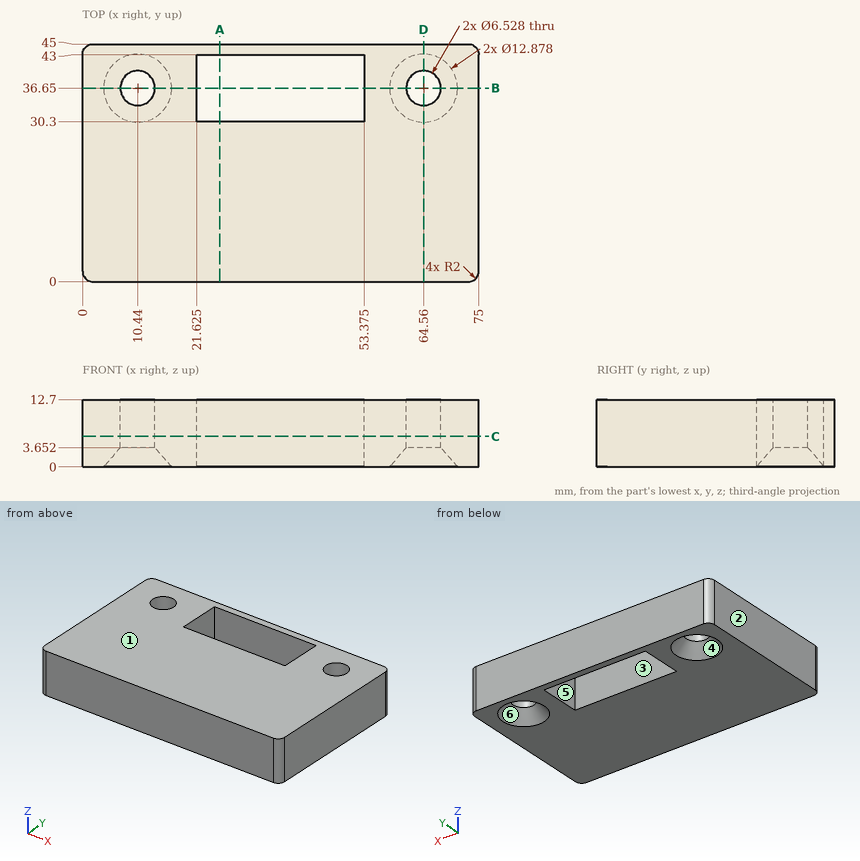
Design review of the part shown in the three views and the two pictorial views. Dimensions are in mm from the part's minimum x, y and z. A direction names the side the tool comes from. Round coordinates to 2 decimals unless told otherwise and drop trailing zeros. Order: outer loops, then holes, each group sorted by start corner. A loop starts at its lowest first (then second) coordinate and runs counter-clockwise, first axis right, second up. Notation, with made-up numbers: (44.25, -9) -> (79.25, -9) arc R18 cw to (79.25, 2) -> close; hole circle Ø8 at (85.25, 59.5). An arc over 180 degrees is marked (long way). Write item = value, one per line. Start each with the question number.
1) Tool access review of the marked faces 5 and 6: name each direction out of +Z, -Z, +X, -X, +Y, -Y from which nothing blocks a thin tool from reaching the whole face with its end or side.
2) Take a section at D-D on x = 64.56. State the section outline as (y, z) points.
3) Insertion check: pin 1 (6 mm diameter, centred on x = 64.56, y = 36.65, fed in from +Z). The pin has a flat end and moves straight along its axis. Give the tip position at first contact, or say it passes through.
4) To check wall thickness, follow line 1 (X direction, y = 36.65, z = 10.75) (1 decimal); line 2 (Y direction, x = 10.44, z = 9); line 3 (Y direction, x = 23, z = 1). State the ranges of each line that lie inside material, in increasing order. Write a range as from..to.
5) Take a section at C-C on z = 5.75. Count the separate pieces of the cut face and the enclosed holes in it, plus the area to 3 significant figures.
6) Take a section at B-B on y = 36.65. State the section outline as (x, z) points (1 decimal).
7) The part is to be moulded in two halves that separate along X. For the marked faces 1, 2, 3 and 4, say which applies: +X half, -X half, draft (parallel to the pull), parting line (faces both ways), or undercut.
8) Take a section at A-A on x = 26. State the section outline as (y, z) points, plus the area to 3 significant figures.
Verdict:
q1.face_5 = +Z, -Z
q1.face_6 = -Z
q2.outline = (0, 0) -> (30.21, 0) -> (33.39, 3.65) -> (33.39, 12.7) -> (0, 12.7) -> close; (39.91, 3.65) -> (43.09, 0) -> (45, 0) -> (45, 12.7) -> (39.91, 12.7) -> close
q3.pin_1 = through
q4.line_1 = 0..7.2, 13.7..21.6, 53.4..61.3, 67.8..75
q4.line_2 = 0..33.39, 39.91..45
q4.line_3 = 0..30.3, 43..45
q5.separate_pieces = 1
q5.enclosed_holes = 3
q5.area = 2,900 mm2
q6.outline = (0, 0) -> (4, 0) -> (7.2, 3.7) -> (7.2, 12.7) -> (0, 12.7) -> close; (13.7, 3.7) -> (16.9, 0) -> (21.6, 0) -> (21.6, 12.7) -> (13.7, 12.7) -> close; (53.4, 0) -> (58.1, 0) -> (61.3, 3.7) -> (61.3, 12.7) -> (53.4, 12.7) -> close; (67.8, 3.7) -> (71, 0) -> (75, 0) -> (75, 12.7) -> (67.8, 12.7) -> close
q7.face_1 = draft
q7.face_2 = -X half
q7.face_3 = undercut
q7.face_4 = undercut
q8.outline = (0, 0) -> (30.3, 0) -> (30.3, 12.7) -> (0, 12.7) -> close; (43, 0) -> (45, 0) -> (45, 12.7) -> (43, 12.7) -> close
q8.area = 410 mm2
